Work out the finished part from the listing and answer in its coordinate system (mm). Coordinates: 2 decimals unless noted, no trailing zeros. Loops run counter-clockwise (first coordinate to the right, second up) from the corner with the lowest first, then second, coordinate; pieces in that order, holes last. Notation, with made-up numbers: (19.25, 14) -> (68.25, 14) arc R21 cw to (68.25, 43) -> close; hole circle Ø3 at (33.25, -20). An arc over 180 degrees is marked (long way). Use a Markdown table: item, result.
Autodesk Inventor part; units mm, degrees
ref_plane "YZ Plane" through (0, 0, 0) normal (1, 0, 0) x (0, 1, 0)
ref_plane "XZ Plane" through (0, 0, 0) normal (0, 1, 0) x (-1, 0, 0)
ref_plane "XY Plane" through (0, 0, 0) normal (0, 0, 1) x (1, 0, 0)
sketch "Sketch1" plane through (0, 0, 0) normal (0, 0, 1) x (1, 0, 0)
  circle A0 centre (0, 0) radius 1.5
  line L0 (0, 0) -> (8, 0)
  circle A1 centre (8, 0) radius 1.5
  line L1 (8, 0) -> (15.5, 0)
  line L2 (15.5, 0) -> (15.5, 4)
  line L3 (15.5, 0) -> (15.5, -4)
  line L4 (15.5, 4) -> (0.8426, 7.1878)
  line L5 (15.5, -4) -> (0.8886, -7.3921)
  line L6 (0, 0) -> (-8, 0)
  line L7 (0.8886, -7.3921) -> (-8, 0)
  line L8 (-8, 0) -> (0.8426, 7.1878)
  dimension "d0" = 3
  dimension "d1" = 8
  dimension "d2" = 3
  dimension "d3" = 7.5
  dimension "d4" = 4
  dimension "d5" = 4
  dimension "d6" = 102.27
  dimension "d7" = 103.07
  dimension "d8" = 15
  dimension "d9" = 15
  dimension "d10" = 8
extrude "Extrusion1" add sketch "Sketch1" against normal blind 16.2 contours L0 A1 L1 L3 L5 L7 L6 A0 | A0 L6 L8 L4 L2 L1 A1 L0
sketch "Sketch2" plane through (0, 0, 0) normal (0, 0, 1) x (1, 0, 0)
  line L0 (15.5, 4) -> (0.8426, 7.1878)
  line L1 (0.8426, 7.1878) -> (-8, 0)
  line L2 (-8, 0) -> (0.8886, -7.3921)
  line L3 (0.8886, -7.3921) -> (15.5, -4)
  line L4 (15.5, -4) -> (15.5, 4)
  circle A0 centre (8, 0) radius 1.5
  circle A1 centre (0, 0) radius 1.5
  line L5 (0.8886, -7.3921) -> (7.7175, -14.6973)
  line L6 (15.5, 4) -> (22.3289, -3.3052)
  arc A2 (41.8621, -51.2233) -> (7.7175, -14.6973) centre (-26.8658, -81.248) ccw
  arc A3 (56.4735, -39.8312) -> (22.3289, -3.3052) centre (-12.2544, -69.8559) ccw
  line L7 (41.8621, -51.2233) -> (53.4151, -60.7903)
  arc A4 (53.4151, -60.7903) -> (63.4535, -48.3329) centre (58.5175, -54.6287) ccw
  line L8 (63.4535, -48.3329) -> (56.4735, -39.8312)
  dimension "d13" = 10
  dimension "d14" = 60
  dimension "d15" = 10
  dimension "d17" = 50
  dimension "d18" = 75
  dimension "d19" = 50
  dimension "d20" = 75
  dimension "d29" = 15
  dimension "d30" = 11
  dimension "d31" = 8
  dimension "d32" = 141.656
extrude "Extrusion2" add sketch "Sketch2" against normal up to surface (16.2 mm away) contours L6 A3 L8 A4 L7 A2 L5 L3 L4
chamfer "Chamfer2" distance 6 angle 45 2 edges at (27.9232, -30.0312, 0) (27.9232, -30.0312, -16.2)
chamfer "Chamfer3" distance 2.5 angle 45 4 edges at (42.5346, -18.6391, -16.2) (42.5346, -18.6391, 0) (22.3289, -3.3052, -8.1) (56.4735, -39.8312, -8.1)
chamfer "Chamfer4" distance 8.5 angle 45 1 edges at (63.4535, -48.3329, -8.1)
chamfer "Chamfer5" distance 2 angle 45 4 edges at (61.1284, -62.1906, 0) (52.1804, -59.7678, 0) (61.1284, -62.1906, -16.2) (52.1804, -59.7678, -16.2)
chamfer "Chamfer6" distance 3 angle 45 1 edges at (66.3346, -56.3297, -8.1)
chamfer "Chamfer7" distance 3 angle 45 1 edges at (-8, 0, -8.1)
properties part number "Tarsus"
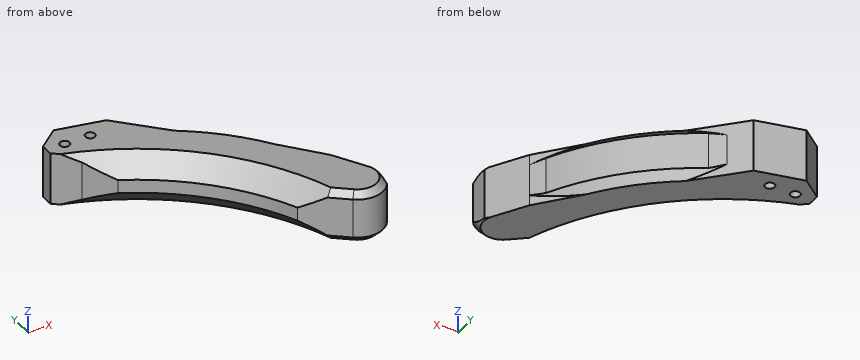
Q1. Consider line 1 (X direction, y = 0, z = -11.5); line 2 (Y direction, x = 0, z = -13); line 3 (Y direction, x = 8, z = -9). Determine where each line is inside the solid, lowest interval first. Write a range as [from, to].
Solved:
| item | result |
|---|---|
| line 1 | [-5.68, -1.5], [1.5, 6.5], [9.5, 19.24] |
| line 2 | [-6.65, -1.5], [1.5, 6.5] |
| line 3 | [-14.84, -1.5], [1.5, 5.63] |
Q2. Section A-A on y = 0 is taken. Determine the outline of the cut face in (x, z), and give its area (3 significant figures).
Solved:
| item | result |
|---|---|
| outline | (-5.68, -16.2) -> (-1.5, -16.2) -> (-1.5, 0) -> (-5.68, 0) -> close; (1.5, -16.2) -> (6.5, -16.2) -> (6.5, 0) -> (1.5, 0) -> close; (9.5, -16.2) -> (19.24, -16.2) -> (19.24, 0) -> (9.5, 0) -> close |
| area | 307 mm² |
Q3. Given pin 1 Ø1.5 at (x, z) = (11.5, -3) entering from -Y; pin 2 Ø6 at (x, z) = (29.5, -11) entering from -Y; pin 3 Ø1.5 at (y, z) = (-7.5, -3.5) entering from +X, each flat-ended and moving along its own axis, determine where each tip first touches the part or whether it passes through.
Solved:
| item | result |
|---|---|
| pin 1 | y = -14.3 |
| pin 2 | y = -35.27 |
| pin 3 | x = 30.52 |
